from build123d import *
from build123d.topology import SkipClean

# Parameters (mm, degrees)
BOSS_EXTRUDE2_DEPTH = 5
CUT_EXTRUDE1_START  = -1
CUT_EXTRUDE1_DEPTH  = 1
CUT_EXTRUDE2_START  = -2
CUT_EXTRUDE2_DEPTH  = 1
CUT_EXTRUDE3_START  = -2
CUT_EXTRUDE3_DEPTH  = 1


with BuildPart() as part:
    # Sketch2 → Boss-Extrude2 (new body)
    with BuildSketch(Plane(origin=(0, 0, 0), x_dir=(1, 0, 0), z_dir=(0, 1, 0))):
        with BuildLine():
            Line((4.85, 2.618089507), (2.8, 2.618089507))
            Line((2.8, 2.618089507), (2.8, 1.224744871))
            Line((2.8, 1.224744871), (1.25, 1.224744871))
            ThreePointArc((1.25, 1.224744871), (-1.728167758, -0.275565237), (1.568910286, -0.775255129))
            Line((1.568910286, -0.775255129), (3.321364344, -0.775255129))
            ThreePointArc((3.321364344, -0.775255129), (17.012963234, -9.713506373), (27.75, 2.618089507))
            Line((27.75, 2.618089507), (25.75, 2.618089507))
            ThreePointArc((25.75, 2.618089507), (15.3, -7.831910493), (4.85, 2.618089507))
        make_face()
    extrude(amount=BOSS_EXTRUDE2_DEPTH)

    # Sketch6 → Cut-Extrude1 (cut)
    with SkipClean():  # the faces are left unmerged after this step: merging them gives an invalid solid
        with BuildSketch(Plane(origin=(0, 5, 0), x_dir=(1, 0, 0), z_dir=(0, 1, 0)).offset(CUT_EXTRUDE1_START)):
            with BuildLine():
                Line((2.8, 1.224744871), (1.25, 1.224744871))
                ThreePointArc((1.25, 1.224744871), (1.728167758, 0.275565237), (1.568910286, -0.775255129))
                Line((1.568910286, -0.775255129), (3.321364344, -0.775255129))
                ThreePointArc((3.321364344, -0.775255129), (3.050160005, 0.22200193), (2.8, 1.224744871))
            make_face()
        extrude(amount=CUT_EXTRUDE1_DEPTH, mode=Mode.SUBTRACT)

    # Sketch8 → Cut-Extrude2 (cut)
    with SkipClean():  # the faces are left unmerged after this step: merging them gives an invalid solid
        with BuildSketch(Plane(origin=(0, 4, 0), x_dir=(1, 0, 0), z_dir=(0, 1, 0)).offset(CUT_EXTRUDE2_START)):
            with BuildLine():
                Line((2.8, 1.224744871), (1.25, 1.224744871))
                ThreePointArc((1.25, 1.224744871), (1.728167758, 0.275565237), (1.568910286, -0.775255129))
                Line((1.568910286, -0.775255129), (3.321364344, -0.775255129))
                ThreePointArc((3.321364344, -0.775255129), (3.050160005, 0.22200193), (2.8, 1.224744871))
            make_face()
        extrude(amount=CUT_EXTRUDE2_DEPTH, mode=Mode.SUBTRACT)

    # Sketch9 → Cut-Extrude3 (cut)
    with SkipClean():  # the faces are left unmerged after this step: merging them gives an invalid solid
        with BuildSketch(Plane(origin=(0, 2, 0), x_dir=(1, 0, 0), z_dir=(0, 1, 0)).offset(CUT_EXTRUDE3_START)):
            with BuildLine():
                Line((2.8, 1.224744871), (1.25, 1.224744871))
                ThreePointArc((1.25, 1.224744871), (1.728167758, 0.275565237), (1.568910286, -0.775255129))
                Line((1.568910286, -0.775255129), (3.321364344, -0.775255129))
                ThreePointArc((3.321364344, -0.775255129), (3.050160005, 0.22200193), (2.8, 1.224744871))
            make_face()
        extrude(amount=CUT_EXTRUDE3_DEPTH, mode=Mode.SUBTRACT)


solid = part.part
Here's how the part is built. I have some questions about the finished solid (model axes, mm). A direction names the side the tool comes from. Give positions to 0.01 mm unless a question says otherwise; leave off trailing zeros. Order: outer loops, then holes, each group sorted by start corner. A loop starts at its lowest first (then second) coordinate and runs counter-clockwise, first axis right, second up. Notation, with made-up numbers: (46.25, 49) -> (50.25, 49) arc R27 ccw to (50.25, 69) -> close; hole circle Ø6 at (62.25, 39). An arc over 180 degrees is marked (long way). One line per item, written item: value. Start each with the question number.
1. We'd pull the mould along X, two halves only. Please class faces 1 (the face through (15.53, 2.46, 7.83)), 2 (the face through (13, 0, 8)): released by +X, released by -X, zero draft, split by the parting line, or undercut.
2. Imagine slicing it at A-A, the plane y = 4.65. List the corners of the cut face in (x, z) for me.
3. Imagine slicing it at C-C, the plane z = 4. List the corners of the cut face in (x, y) for me.
4. I need wall thicknesses on probe 1 along X at (y, z) = (4.4, -1); probe 2 along X at (y, z) = (4.3, -0.5); probe 3 along X at (y, z) = (1.4, 2.5). Which ranges of each line are inside material? Lowest first, please. Write a range as from..to.
5. Imagine slicing it at B-B, the plane z = 0. List the corners of the cut face in (x, y) for me, plus the area to 3 significant figures.
6. For faces 3 (the face through (2, 3.5, -1.225)), 4 (the face through (3.054, 2.493, -0.208)), 5 (the face through (3.054, 0.493, -0.208)), 6 (the face through (2.4, 3.5, 0.775)), which set-ups out of +Z, -Z, +X, -X, +Y, -Y let a thin tool reach every point of the face, with its end or its side?
7. Imagine slicing it at D-D, the plane x = 0. List the corners of the cut face in (y, z) for me.
8. Will these pins go through, and if not, where does the flat tip stop? pin 1 Ø1.6 at (x, z) = (2.5, -0.5) entering from -Y; pin 2 Ø1 at (x, y) = (8, 4.5) entering from -Z; pin 3 Ø1.5 at (y, z) = (2, 4.5) entering from +X; pin 4 Ø0.8 at (x, y) = (2.5, 1.5) entering from +Z.
Values follow:
1. face 1: undercut
1. face 2: zero draft
2. outline: circle Ø3.5 at (0, 0); (2.8, -2.62) -> (4.85, -2.62) arc R10.45 cw to (25.75, -2.62) -> (27.75, -2.62) arc R12.45 ccw to (3.32, 0.78) arc R49.11 ccw to (2.8, -1.22) -> close
3. outline: (4.75, 0) -> (7.21, 0) -> (7.21, 5) -> (4.75, 5) -> close; (23.39, 0) -> (25.85, 0) -> (25.85, 5) -> (23.39, 5) -> close
4. probe 1: x = -1.44..1.44, 2.85..4.98, 25.62..27.64
4. probe 2: x = -1.68..1.68, 2.98..5.07, 25.53..27.57
4. probe 3: x = 3.95..6.19, 24.41..26.65
5. outline: (-1.75, 0) -> (1.75, 0) -> (1.75, 1) -> (3.11, 1) -> (3.11, 0) -> (5.18, 0) -> (5.18, 5) -> (3.11, 5) -> (3.11, 4) -> (1.75, 4) -> (1.75, 5) -> (-1.75, 5) -> close; (25.42, 0) -> (27.47, 0) -> (27.47, 5) -> (25.42, 5) -> close; hole (1.75, 2) -> (3.11, 2) -> (3.11, 3) -> (1.75, 3) -> close
5. area: 40.9 mm2
6. face 3: -Z, +Y, -Y
6. face 4: +Z
6. face 5: +Z, -Y
6. face 6: +Z, +Y, -Y
7. outline: (0, -1.75) -> (5, -1.75) -> (5, 1.75) -> (0, 1.75) -> close
8. pin 1: stops at y = 0
8. pin 2: stops at z = 4.34
8. pin 3: stops at x = 26
8. pin 4: stops at z = 0.78
